```python
from build123d import *

# Parameters (mm, degrees)
EXTRUDE_1_DEPTH     = 80
SKETCH_2_R          = 3
EXTRUDE_2_DEPTH     = 8
SKETCH_3_R          = 3
CUT_EXTRUDE_1_DEPTH = 8


with BuildPart() as part:
    # 草图1 → 凸台-拉伸1 (new body)
    with BuildSketch(Plane(origin=(0, 0, 0), x_dir=(1, 0, 0), z_dir=(0, 1, 0))):
        Polygon((4.610693432, 8.004676097), (-4.626906133, 7.995315689), (-9.237599565, -0.009360407), (-4.610693432, -8.004676097), (4.626906133, -7.995315689), (9.237599565, 0.009360407), align=None)
    extrude(amount=EXTRUDE_1_DEPTH)

    # 草图2 → 凸台-拉伸2 (add)
    with BuildSketch(Plane(origin=(0, 80, 0), x_dir=(1, 0, 0), z_dir=(0, 1, 0))):
        Circle(SKETCH_2_R)
    extrude(amount=EXTRUDE_2_DEPTH)

    # 草图3 → 切除-拉伸1 (cut)
    with BuildSketch(Plane.XZ):
        Circle(SKETCH_3_R)
    extrude(amount=-CUT_EXTRUDE_1_DEPTH, mode=Mode.SUBTRACT)


solid = part.part
```
Model file for the job. Use its own axes, mm. A direction names the side the tool comes from. Coordinates: 2 decimals unless noted, no trailing zeros. Loops run counter-clockwise (first coordinate to the right, second up) from the corner with the lowest first, then second, coordinate; pieces in that order, holes last. Notation, with made-up numbers: (8.5, 31.5) -> (33.5, 31.5) arc R20 cw to (33.5, 69.5) -> close; hole circle Ø1 at (8, 18). An arc over 180 degrees is marked (long way). Answer as a JSON object with one key per item and string values.
Q1. Cut at D-D (z = 7). List the corners of the cut face in (x, y).
Report:
{"outline": "(-5.19, 0) -> (5.2, 0) -> (5.2, 80) -> (-5.19, 80) -> close"}
Q2. Flat gauge pins, fed straight in: P1, Ø6, axis at x = 4, z = 4, coming from the +Y side; P2, Ø6, axis at x = -7, z = 0.5, coming from the +Y side; P3, Ø1.8, axis at x = 0, z = -1.5, coming from the -Y side; P4, Ø4, axis at y = 21.5, z = 0.5, coming from the +X side. Where does each tip first touch, or does it go through?
Report:
{"P1": "stops at y = 88", "P2": "stops at y = 80", "P3": "stops at y = 8", "P4": "stops at x = 9.24"}
Q3. Probe probe 1 along Z at (x, y) = (0, 5.5); probe 2 along Y at (x, z) = (-5.75, 5.75); probe 3 along Z at (x, y) = (1.25, 74). List the from-to ranges inside material, lowest first.
Report:
{"probe 1": "z = -8 to -3, 3 to 8", "probe 2": "y = 0 to 80", "probe 3": "z = -8 to 8"}
Q4. Pull direction X, two halves, no side cores. Call faces 1 (the cylindrical face through (-3, 4, 0)), 2 (the flat face through (0, 8, 0)), 3 (the flat face through (6.9, 39.44, 4.05)), 4 (the flat face through (4, 0, 0)): released by +X, released by -X, zero draft, split by the parting line, or undercut.
Report:
{"face 1": "undercut", "face 2": "undercut", "face 3": "released by +X", "face 4": "zero draft"}
Q5. Cut at C-C (z = 1.5). List the corners of the cut face in (x, y), and give its area (3 significant figures).
Report:
{"outline": "(-8.37, 0) -> (-2.6, 0) -> (-2.6, 8) -> (2.6, 8) -> (2.6, 0) -> (8.37, 0) -> (8.37, 80) -> (2.6, 80) -> (2.6, 88) -> (-2.6, 88) -> (-2.6, 80) -> (-8.37, 80) -> close", "area": "1,340 mm2"}
Q6. Cut at A-A (x = 0). List the corners of the cut face in (y, z).
Report:
{"outline": "(0, -8) -> (80, -8) -> (80, -3) -> (88, -3) -> (88, 3) -> (80, 3) -> (80, 8) -> (0, 8) -> (0, 3) -> (8, 3) -> (8, -3) -> (0, -3) -> close"}
Q7. Cut at B-B (y = 43). List the corners of the cut face in (x, z), and give its area (3 significant figures).
Report:
{"outline": "(-9.24, 0.01) -> (-4.63, -8) -> (4.61, -8) -> (9.24, -0.01) -> (4.63, 8) -> (-4.61, 8) -> close", "area": "222 mm2"}
Q8. 3-axis set-ups, long thin cutter, end or side, ignore diameter. For faces 5 (the flat face through (4, 80, 0)), 6 (the flat face through (-6.9, 39.44, -4.05)): which of +Z, -Z, +X, -X, +Y, -Y reach the whole face in a straight line?
Report:
{"face 5": "+Y", "face 6": "-Z, -X, +Y, -Y"}
